from build123d import *

# Parameters (mm, degrees)
F0_R     = 10
F1_DEPTH = 40
F0_R_2   = 30
F2_DEPTH = 120
F0_R_3   = 50
F3_DEPTH = 140


with BuildPart() as f1:
    # F0 (on Front) → F1 (new body)
    with BuildSketch(Plane.XZ):
        with Locations((0.03067, 0)):
            Circle(F0_R)
    extrude(amount=F1_DEPTH)

    # F0 (on Front) → F2 (join)
    with BuildSketch(Plane.XZ):
        Circle(F0_R_2)
        with Locations((0.03067, 0)):
            Circle(F0_R, mode=Mode.SUBTRACT)
    extrude(amount=F2_DEPTH)

    # F0 (on Front) → F3 (join)
    with BuildSketch(Plane.XZ):
        with Locations((0.03067, 0)):
            Circle(F0_R_3)
        Circle(F0_R_2, mode=Mode.SUBTRACT)
    extrude(amount=F3_DEPTH)


solid = f1.part
Source: CAD feature listing. Evaluate the final solid. Frame: model axes, mm. A direction names the side the tool comes from. Give positions to 0.01 mm unless a question says otherwise; leave off trailing zeros. Write each loop counter-clockwise with the first axis right and the second up, starting at its lowest first coordinate (ties: lowest second). Pieces come first, ordered by that corner, then holes. Notation, with made-up numbers: (73, 76.5) -> (87, 76.5) arc R19 ccw to (87, 100.5) -> close; hole circle Ø7 at (-19, -28). An arc over 180 degrees is marked (long way). Return JSON: item names as keys, results as strings. Group by question number.
1. Section C-C, the plane x = 5.5. Output: boundary loops of the cut face in (y, z), then the cut area to 3 significant figures.
2. Access query for faces 1 (the face through (13, -120, 0)), 2 (the face through (22, -140, -22)). Directions: +Z, -Z, +X, -X, +Y, -Y. A direction counts if a zero-diameter tool reaches every point of the face in a straight line with its end or side. Return the directions, or none.
3. Pin query (flat end, axial travel): pin 1 Ø6 at (x, z) = (2.5, 2) entering from -Y; pin 2 Ø5 at (x, y) = (-10, -110) entering from -Z; pin 3 Ø18 at (x, z) = (-9.5, -4.5) entering from -Y. Return the tip coordinate at first contact, or that it passes through.
4. Section A-A, the plane y = -127.5. Output: boundary loops of the cut face in (x, z).
5. Mould query, pull axis Z, two halves, no side actions, for faces 3 (the face through (47.72, -69.02, 15.02)), 4 (the face through (0, -40, 0)), 5 (the face through (-1, 0, 1)). Classes: +Z half, -Z half, draft (parallel to the pull), parting line (faces both ways), or undercut.
6. Section D-D, the plane y = -76. Output: boundary loops of the cut face in (x, z), then the cut area to 3 significant figures.
7. Material intervals for line 1 (Y direction, x = -10.5, z = 2); line 2 (X direction, y = -126.5, z = -27.5); line 3 (Z direction, x = -6, y = -110), sorted ascending. Write a range as from..to.
8. Section B-B, the plane z = 0. Output: boundary loops of the cut face in (x, y).
Determined:
{
 "1": {"outline": "(-140, -49.7) -> (0, -49.7) -> (0, 49.7) -> (-140, 49.7) -> (-140, 29.49) -> (-120, 29.49) -> (-120, 8.37) -> (-40, 8.37) -> (-40, -8.37) -> (-120, -8.37) -> (-120, -29.49) -> (-140, -29.49) -> close", "area": "11,400 mm2"},
 "2": {"face 1": "-Y", "face 2": "+Z, -Z, +X, -X, -Y"},
 "3": {"pin 1": "stops at y = -40", "pin 2": "stops at z = -49.43", "pin 3": "stops at y = -120"},
 "4": {"outline": "circle Ø100 at (0.03, 0); hole circle Ø60 at (0, 0)"},
 "5": {"face 3": "parting line", "face 4": "undercut", "face 5": "draft"},
 "6": {"outline": "circle Ø100 at (0.03, 0); hole circle Ø20 at (0.03, 0)", "area": "7,540 mm2"},
 "7": {"line 1": "y = -120..0", "line 2": "x = -41.73..-11.99, 11.99..41.79", "line 3": "z = -49.63..-7.98, 7.98..49.63"},
 "8": {"outline": "(-49.97, -140) -> (-30, -140) -> (-30, -120) -> (-9.97, -120) -> (-9.97, -40) -> (10.03, -40) -> (10.03, -120) -> (30, -120) -> (30, -140) -> (50.03, -140) -> (50.03, 0) -> (-49.97, 0) -> close"}
}
